Build history of the part. All positions in model axes, mm. A direction names the side the tool comes from. Give positions to 0.01 mm unless a question says otherwise; leave off trailing zeros. Order: outer loops, then holes, each group sorted by start corner. A loop starts at its lowest first (then second) coordinate and runs counter-clockwise, first axis right, second up. Notation, with made-up numbers: (-10, -18) - (48, -18) arc R20 ccw to (48, 17) - close; hole circle Ø3 at (8.25, 63). An arc over 180 degrees is marked (long way). Use a Markdown table: item, result. Add a question column.
(1) Flat gauge pins, fed straight in: pin 1 (2 mm diameter, centred on y = 140, z = -738.5, fed in from -X); pin 2 (10 mm diameter, centred on x = 77, y = 151, fed in from +Z); pin 3 (12 mm diameter, centred on x = -478.5, z = -785, fed in from +Y); pin 4 (12 mm diameter, centred on y = 212.5, z = -666.5, fed in from +X). Where does each tip first touch, or does it go through?
(2) Which spindle directions (+Z, -Z, +X, -X, +Y, -Y) get a long thin tool onto all of the face, cutting with end or side? Do faces 1 (the face through (-603.25, 10, -706)), 2 (the face through (-0.42, 178.58, -791.34)), 3 (the face through (411, 20, -623)). Say none if no direction does.
(3) Slice it at D-D (z = -760.5). Write the cut outline in (x, y).
(4) Slice it at C-C (z = -666). Write the cut outline in (x, y).
(5) Mould opens along X. For faces 4 (the face through (-117.14, 212.176, -704.887)), 5 (the face through (623.25, 10, -706)), 6 (the face through (30, 134, -706)) say: +X half, -X half, draft (parallel to the pull), parting line (faces both ways), or undercut.
(6) Slice it at B-B (x = 372.5). Write the cut outline in (y, z).
(7) Wall check: line 1 (X direction, y = 161, z = -631); line 2 (X direction, y = 109.5, z = -622); line 3 (Y direction, x = 47.5, z = -617.5). Give the ranges that are in metal, low to high.
(8) Slice it at A-A (y = 53). Write the cut outline in (x, z).
from build123d import *

# Parameters (mm, degrees)
BOSS_EXTRUDE1_DEPTH      = 20
SKETCH2_W                = 254
SKETCH2_H                = 207.844806097
BOSS_EXTRUDE2_DEPTH      = 20
SKETCH3_R                = 10
BOSS_EXTRUDE3_DEPTH      = 20
BOSS_EXTRUDE4_DEPTH      = 30
BOSS_EXTRUDE4_DEPTH_BACK = 30
SKETCH4_R                = 88.24460582
SKETCH5_R                = 10
BOSS_EXTRUDE5_DEPTH      = 254


with BuildPart() as part:
    # Sketch1 → Boss-Extrude1 (new body)
    with BuildSketch(Plane(origin=(0, 0, 0), x_dir=(1, 0, 0), z_dir=(0, 1, 0))):
        Polygon((-623.25, 811.094806097), (-623.25, 623.25), (-603.25, 623.25), (-603.25, 791.094806097), (603.25, 791.094806097), (603.25, 623.25), (623.25, 623.25), (623.25, 811.094806097), align=None)
        Polygon((-623.25, 623.25), (-623.25, 603.25), (-603.25, 603.25), (603.25, 603.25), (623.25, 603.25), (623.25, 623.25), (603.25, 623.25), (-603.25, 623.25), align=None)
    extrude(amount=BOSS_EXTRUDE1_DEPTH)

    # Sketch2 → Boss-Extrude2 (add)
    with BuildSketch(Plane(origin=(0, 20, 0), x_dir=(1, 0, 0), z_dir=(0, 1, 0))):
        with Locations((0, 707.172403048)):
            Rectangle(SKETCH2_W, SKETCH2_H)
    extrude(amount=BOSS_EXTRUDE2_DEPTH)

    # Sketch3 → Boss-Extrude3 (add)
    with BuildSketch(Plane.ZY.offset(127)):
        with BuildLine():
            Line((-811.094806097, 40), (-603.25, 40))
            Line((-603.25, 40), (-603.25, 108.279126424))
            ThreePointArc((-603.25, 108.279126424), (-707.172403048, 212.201529473), (-811.094806097, 108.279126424))
            Line((-811.094806097, 108.279126424), (-811.094806097, 40))
        make_face()
        with Locations((-707.172403048, 152.06935065)):
            Circle(SKETCH3_R, mode=Mode.SUBTRACT)
    boss_extrude3 = extrude(amount=-BOSS_EXTRUDE3_DEPTH)

    # Mirror1: Boss-Extrude3 across plane
    add(boss_extrude3.mirror(Plane(origin=(0, 0, 0), x_dir=(0, 0, 1), z_dir=(1, 0, 0))))



with BuildPart() as body_2:
    # Sketch4 → Boss-Extrude4 (new, two sides: drawn at the far end of the back side and taken through both)
    with BuildSketch(Plane(origin=(0, 0, 0), x_dir=(0, 0, -1), z_dir=(1, 0, 0)).offset(-BOSS_EXTRUDE4_DEPTH_BACK)):
        with Locations((707.172403048, 152.06935065)):
            Circle(SKETCH4_R)
    extrude(amount=BOSS_EXTRUDE4_DEPTH + BOSS_EXTRUDE4_DEPTH_BACK)


with BuildPart() as part_1:
    add(part.part)

    add(body_2.part)  # Boss-Extrude5 merges body 2
    # Sketch5 → Boss-Extrude5 (add)
    with BuildSketch(Plane.ZY.offset(127)):
        with Locations(Location((-707.172403048, 152.06935065, 0), (0, 0, 180))):
            Circle(SKETCH5_R)
    extrude(amount=-BOSS_EXTRUDE5_DEPTH)


solid = part_1.part
Solution:
| question | item | result |
|---|---|---|
| 1 | pin 1 | x = -127 |
| 1 | pin 2 | z = -697.17 |
| 1 | pin 3 | through |
| 1 | pin 4 | x = 30 |
| 2 | face 1 | +Y, -Y |
| 2 | face 2 | none |
| 2 | face 3 | +Z, -Z, +X, +Y |
| 3 | outline | (-623.25, 0) - (-603.25, 0) - (-603.25, 20) - (-623.25, 20) - close; (-127, 20) - (127, 20) - (127, 197.48) - (107, 197.48) - (107, 40) - (-107, 40) - (-107, 197.48) - (-127, 197.48) - close; (-30, 81.76) - (30, 81.76) - (30, 222.38) - (-30, 222.38) - close; (603.25, 0) - (623.25, 0) - (623.25, 20) - (603.25, 20) - close |
| 4 | outline | (-623.25, 0) - (-603.25, 0) - (-603.25, 20) - (-623.25, 20) - close; (-127, 20) - (127, 20) - (127, 203.7) - (107, 203.7) - (107, 40) - (-107, 40) - (-107, 203.7) - (-127, 203.7) - close; (-30, 74.02) - (30, 74.02) - (30, 230.12) - (-30, 230.12) - close; (603.25, 0) - (623.25, 0) - (623.25, 20) - (603.25, 20) - close |
| 5 | face 4 | draft |
| 5 | face 5 | +X half |
| 5 | face 6 | undercut |
| 6 | outline | (0, -811.09) - (20, -811.09) - (20, -791.09) - (0, -791.09) - close; (0, -623.25) - (20, -623.25) - (20, -603.25) - (0, -603.25) - close |
| 7 | line 1 | -127 to -107, -30 to 30, 107 to 127 |
| 7 | line 2 | -127 to -107, 107 to 127 |
| 7 | line 3 | 0 to 40 |
| 8 | outline | (-127, -811.09) - (-107, -811.09) - (-107, -603.25) - (-127, -603.25) - close; (107, -811.09) - (127, -811.09) - (127, -603.25) - (107, -603.25) - close |
